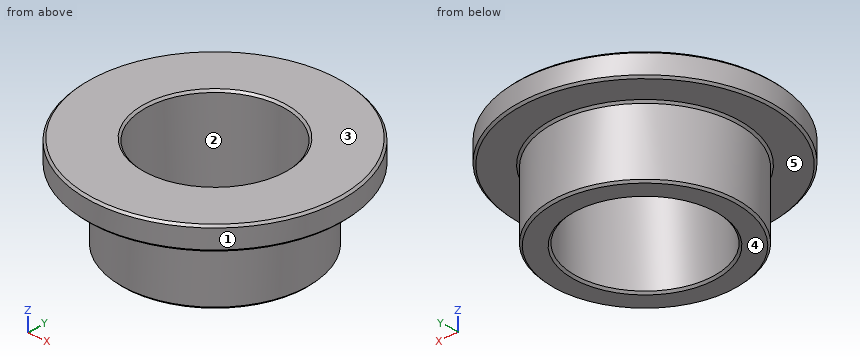
```python
from build123d import *

# Parameters (mm, degrees)
BOSS_EXTRUDE1_START = 3.175
SKETCH3_R           = 8.73125
SKETCH3_R_2         = 4.7752
BOSS_EXTRUDE1_DEPTH = 1.5875
BOSS_EXTRUDE2_START = 1.5875
SKETCH4_R           = 6.3754
SKETCH4_R_2         = 4.7752
BOSS_EXTRUDE2_DEPTH = 4.7625
CHAMFER1_SIZE       = 0.143256


with BuildPart() as part:
    # Sketch3 → Boss-Extrude1 (new body)
    with BuildSketch(Plane.XY.offset(BOSS_EXTRUDE1_START)):
        Circle(SKETCH3_R)
        Circle(SKETCH3_R_2, mode=Mode.SUBTRACT)
    extrude(amount=-BOSS_EXTRUDE1_DEPTH)

    # Sketch4 → Boss-Extrude2 (add)
    with BuildSketch(Plane.XY.offset(BOSS_EXTRUDE2_START)):
        Circle(SKETCH4_R)
        Circle(SKETCH4_R_2, mode=Mode.SUBTRACT)
    extrude(amount=-BOSS_EXTRUDE2_DEPTH)

    # Chamfer1
    chamfer1_edges = [part.edges().sort_by_distance(p)[0] for p in [
        (-4.7752, 0, -3.175),
        (-6.3754, 0, 1.5875),
        (-8.73125, 0, 3.175),
        (-8.73125, 0, 1.5875),
        (-4.7752, 0, 3.175),
        (-6.3754, 0, -3.175),
    ]]
    chamfer(chamfer1_edges, length=CHAMFER1_SIZE)


solid = part.part
```
Design review of the part built by this model. Coordinates are the model's own, in mm. Face numbers are marked on the shaded views. A direction names the side the tool comes from. Round coordinates to 2 decimals unless told otherwise and drop trailing zeros. Write each loop counter-clockwise with the first axis right and the second up, starting at its lowest first coordinate (ties: lowest second). Pieces come first, ordered by that corner, then holes. Notation, with made-up numbers: (75, 69) -> (119, 69) arc R18 ccw to (119, 97) -> close; hole circle Ø6 at (14, -33.5). An arc over 180 degrees is marked (long way). Answer in a Markdown table with one row per item.
Q1. Take a section at C-C, the plane z = -1.5. State the section outline as (x, y) points, then the cut area to 3 significant figures.
The answers:
| item | result |
|---|---|
| outline | circle Ø12.75 at (0, 0); hole circle Ø9.55 at (0, 0) |
| area | 56.1 mm² |
Q2. Draft analysis for pull direction X (two halves, no side actions). For the marked faces 1, 2 and 3, state which applies: +X half, -X half, draft (parallel to the pull), parting line (faces both ways), or undercut.
The answers:
| item | result |
|---|---|
| face 1 | parting line |
| face 2 | undercut |
| face 3 | draft |
Q3. Take a section at D-D, the plane z = 2.75. State the section outline as (x, y) points, then the cut area to 3 significant figures.
The answers:
| item | result |
|---|---|
| outline | circle Ø17.46 at (0, 0); hole circle Ø9.55 at (0, 0) |
| area | 168 mm² |
Q4. To check wall thickness, follow L1, parallel to Y at x = 0, z = 1.25; L2, parallel to Y at x = -1.5, z = 1.25; L3, parallel to Z at x = 6.75, y = -3.5 (1 decimal). State the ranges of each line that lie inside material, in increasing order. Write a range as [from, to].
The answers:
| item | result |
|---|---|
| L1 | [-6.38, -4.78], [4.78, 6.38] |
| L2 | [-6.2, -4.53], [4.53, 6.2] |
| L3 | [1.6, 3.2] |
Q5. Clearance check with flat-ended pins moving along their axes: pin 1 Ø10 at (x, y) = (-2, -2) entering from +Z (3 decimals); pin 2 Ø2 at (x, z) = (5.5, 0) entering from +Y. State where each tip first meets the part, or that it passes through.
The answers:
| item | result |
|---|---|
| pin 1 | z = 3.175 |
| pin 2 | y = 4.52 |
Q6. For the marked faces 4 and 5, list the 3-axis set-ups (+Z, -Z, +X, -X, +Y, -Y) from which the entire face can be reached by the end or side of a thin tool; tool diameter is ignored.
The answers:
| item | result |
|---|---|
| face 4 | -Z, +X, -X, +Y, -Y |
| face 5 | -Z |
